```python
from build123d import *

# Parameters (mm, degrees)
SKETCH_1_R          = 0.5
SKETCH_1_R_2        = 0.4
SKETCH_1_R_3        = 0.425
EXTRUDE_1_DEPTH     = 0.5
SKETCH_2_R          = 4.472023715
CUT_EXTRUDE_1_DEPTH = 0.1
SKETCH_3_R          = 0.7
CUT_EXTRUDE_2_DEPTH = 0.35
SKETCH_4_R          = 4.472023715
SKETCH_4_R_2        = 1
CUT_EXTRUDE_3_DEPTH = 0.05
FILLET_1_R          = 0.1
SKETCH_5_R          = 0.6
CUT_EXTRUDE_4_DEPTH = 10


with BuildPart() as part:
    # Эскиз1 → Бобышка-Вытянуть1 (new body)
    with BuildSketch(Plane.XY):
        with BuildLine():
            Line((12.966197468, 6.264002172), (12.290985741, 6.014467613))
            ThreePointArc((12.290985741, 6.014467613), (9.503979032, 5.15824387), (8.79665468, 2.329778252))
            ThreePointArc((8.79665468, 2.329778252), (7.979149058, 1.075012683), (6.832886069, 2.038772631))
            ThreePointArc((6.832886069, 2.038772631), (4.771275566, 6.759132651), (0, 8.7))
            ThreePointArc((0, 8.7), (-6.815908497, 5.406791226), (-8.471768795, -1.979680148))
            ThreePointArc((-8.471768795, -1.979680148), (-10.930300525, -1.329835953), (-13.004676896, 0.141095189))
            ThreePointArc((-13.004676896, 0.141095189), (-12.194658567, 2.119542362), (-12.085233501, 4.254585469))
            ThreePointArc((-12.085233501, 4.254585469), (-12.076804664, 4.545349887), (-11.984771054, 4.821293371))
            Line((-11.984771054, 4.821293371), (-8.849528074, 11.018100783))
            ThreePointArc((-8.849528074, 11.018100783), (-8.490551174, 11.546729856), (-8.009291923, 11.967089993))
            ThreePointArc((-8.009291923, 11.967089993), (3.778098837, 13.895537743), (12.966197468, 6.264002172))
        make_face()
        with Locations((7.832562474, 2.064210526)):
            Circle(SKETCH_1_R, mode=Mode.SUBTRACT)
        with Locations((0, 9.5)):
            Circle(SKETCH_1_R, mode=Mode.SUBTRACT)
        with Locations((-10.935928421, 0.135601584)):
            Circle(SKETCH_1_R_2, mode=Mode.SUBTRACT)
        with Locations((-9.112495388, 6.401403857)):
            Circle(SKETCH_1_R_3, mode=Mode.SUBTRACT)
        with Locations((7.411343366, 9.626689996)):
            Circle(SKETCH_1_R_3, mode=Mode.SUBTRACT)
        with Locations((10.679257851, 8.251019039)):
            Circle(SKETCH_1_R_2, mode=Mode.SUBTRACT)
    extrude(amount=EXTRUDE_1_DEPTH)

    # Эскиз2 → Вырез-Вытянуть1 (cut)
    with BuildSketch(Plane(origin=(0, 0, 0), x_dir=(-1, 0, 0), z_dir=(0, 0, -1))):
        with Locations((-7.832562474, 2.064210526)):
            Circle(SKETCH_2_R)
    extrude(amount=-CUT_EXTRUDE_1_DEPTH, mode=Mode.SUBTRACT)

    # Эскиз3 → Вырез-Вытянуть2 (cut)
    with BuildSketch(Plane.XY.offset(0.5)):
        with Locations((-9.112495388, 6.401403857)):
            Circle(SKETCH_3_R)
        with Locations((7.411343366, 9.626689996)):
            Circle(SKETCH_3_R)
    extrude(amount=-CUT_EXTRUDE_2_DEPTH, mode=Mode.SUBTRACT)

    # Эскиз4 → Вырез-Вытянуть3 (cut)
    with BuildSketch(Plane(origin=(0, 0, 0.1), x_dir=(-1, 0, 0), z_dir=(0, 0, -1))):
        with Locations((-7.832562474, 2.064210526)):
            Circle(SKETCH_4_R)
        with Locations((-7.832562474, 2.064210526)):
            Circle(SKETCH_4_R_2, mode=Mode.SUBTRACT)
    extrude(amount=-CUT_EXTRUDE_3_DEPTH, mode=Mode.SUBTRACT)

    # Скругление1
    fillet_1_edges = [part.edges().sort_by_distance(p)[0] for p in [
        (12.966197468, 6.264002172, 0.25),
        (12.290985741, 6.014467613, 0.25),
        (-8.471768795, -1.979680148, 0.25),
        (-13.004676896, 0.141095189, 0.25),
        (10.333057023, 5.771840917, 0.075),
        (5.521987637, 5.893079815, 0.075),
    ]]
    fillet(fillet_1_edges, radius=FILLET_1_R)

    # Эскиз5 → Вырез-Вытянуть4 (cut)
    with BuildSketch(Plane.XY.offset(0.5)):
        with Locations((-11.09555803, 4.371400595)):
            Circle(SKETCH_5_R)
        with Locations((11.442307716, 7.164048725)):
            Circle(SKETCH_5_R)
        with Locations((-1.336244315, 13.433705785)):
            Circle(SKETCH_5_R)
    extrude(amount=-CUT_EXTRUDE_4_DEPTH, mode=Mode.SUBTRACT)


solid = part.part
```
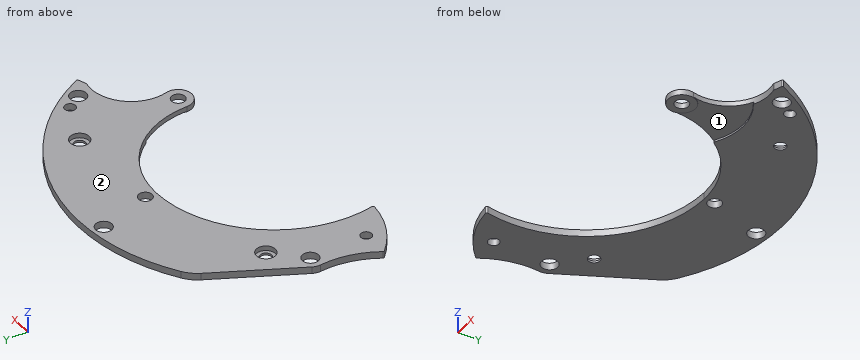
Source: CAD feature listing. Evaluate the final solid. Frame: model axes, mm. Face numbers are marked on the shaded views. Round coordinates to 2 decimals unless told otherwise and drop trailing zeros. Loops run counter-clockwise (first coordinate to the right, second up) from the corner with the lowest first, then second, coordinate; pieces in that order, holes last. Notation, with made-up numbers: (36.25, -20) - (68.25, -20) arc R27 ccw to (68.25, -4) - close; hole circle Ø10 at (-24.75, 20). An arc over 180 degrees is marked (long way). Use CSV: the item, a comma, the result in double quotes.
Q1. Section query C-C, the plane x = 6. Output: boundary loops of the cut face in (y, z).
Reported:
outline,"(5.14, 0.15) - (6.14, 0.15) - (6.14, 0) - (13.09, 0) - (13.09, 0.5) - (5.14, 0.5) - close"
Q2. Mould query, pull axis X, two halves, no side actions, for the marked faces 1 and 2. Classes: pulls with the +X half, pulls with the -X half, needs draft (parallel to the pull), parting line crosses it, or undercut.
Reported:
face 1,"undercut"
face 2,"needs draft"
Q3. Section query A-A, the plane z = 0.3. Give the number of separate pieces and of enclosed holes in the cut face, then the cut area to 3 significant figures.
Reported:
separate pieces,"1"
enclosed holes,"9"
area,"163 mm^2"
Q4. Section query B-B, the plane x = 1.5. Output: boundary loops of the cut face in (y, z), then the cut area to 3 significant figures.
Reported:
outline,"(8.53, 0) - (14.32, 0) - (14.32, 0.5) - (8.53, 0.5) - close"
area,"2.89 mm^2"
Q5. Pin query (flat end, axial travel): pin 1 Ø0.7 at (x, y) = (-1.34, 13.43) entering from +Z; pin 2 Ø1.6 at (x, y) = (7.5, 2) entering from -Z; pin 3 Ø2 at (x, y) = (7, 4) entering from -Z. Return the tip coordinate at first contact, or that it passes through.
Reported:
pin 1,"through"
pin 2,"z = 0.1"
pin 3,"z = 0.15"
Q6. Ray query, line 1 along X through (y, z) = (4.5, 0.4); line 2 along Y through (x, z) = (0, 0.3); line 3 along X through (y, z) = (4.75, 0.45). Return the intervals inside material, ascending.
Reported:
line 1,"-12.08 to -11.68, -10.51 to -7.45, 6.31 to 9.03"
line 2,"8.7 to 9, 10 to 14.4"
line 3,"-12.02 to -11.56, -10.63 to -7.29, 6.2 to 9.18"
